Check sheet for the modelled part. Datum: model origin and axes. Units: mm. A direction names the side the tool comes from. Coordinates: 2 decimals unless noted, no trailing zeros. Write each loop counter-clockwise with the first axis right and the second up, starting at its lowest first coordinate (ties: lowest second). Pieces come first, ordered by that corner, then holes. Notation, with made-up numbers: (-1.5, 63.5) - (10.5, 63.5) arc R36 cw to (10.5, 101.5) - close; hole circle Ø11 at (73, 88.25). An arc over 180 degrees is marked (long way). Answer as CSV lines item,"result". Start each with the question number.
Autodesk Inventor part; units mm, degrees
ref_plane "YZ Plane" through (0, 0, 0) normal (1, 0, 0) x (0, 1, 0)
ref_plane "XZ Plane" through (0, 0, 0) normal (0, 1, 0) x (-1, 0, 0)
ref_plane "XY Plane" through (0, 0, 0) normal (0, 0, 1) x (1, 0, 0)
sketch "スケッチ1" plane through (0, 0, 0) normal (0, 0, 1) x (1, 0, 0)
  line L0 (-28, 65) -> (28, 65)
  line L1 (28, 65) -> (28, 47.1)
  line L2 (-28, -65) -> (-28, -47.1)
  line L3 (-28, 65) -> (28, -65) construction
  line L4 (28, 65) -> (-28, -65) construction
  line L5 (-28, 45) -> (-33, 45)
  line L6 (-33, 15) -> (-28, 15)
  line L7 (-33, 15) -> (-33, 45)
  line L8 (-28, -15) -> (-33, -15)
  line L9 (-33, -15) -> (-33, -45)
  line L10 (-33, -45) -> (-28, -45)
  arc A0 (-28, 45) -> (-28, 47.1) centre (-28, 46.05) ccw
  arc A1 (-28, 12.9) -> (-28, 15) centre (-28, 13.95) ccw
  arc A2 (-28, -15) -> (-28, -12.9) centre (-28, -13.95) ccw
  arc A3 (-28, -47.1) -> (-28, -45) centre (-28, -46.05) ccw
  line L11 (-28, 47.1) -> (-28, 65)
  line L12 (-28, 12.9) -> (-28, 15) construction
  line L13 (-28, -12.9) -> (-28, 12.9)
  line L14 (-28, -47.1) -> (-28, -45) construction
  line L15 (0, 65) -> (0, -65) construction
  arc A4 (28, -45) -> (28, -47.1) centre (28, -46.05) ccw
  line L16 (33, -45) -> (28, -45)
  line L17 (33, -15) -> (33, -45)
  line L18 (28, -15) -> (33, -15)
  arc A5 (28, -12.9) -> (28, -15) centre (28, -13.95) ccw
  arc A6 (28, 15) -> (28, 12.9) centre (28, 13.95) ccw
  line L19 (33, 15) -> (33, 45)
  line L20 (33, 15) -> (28, 15)
  line L21 (28, 45) -> (33, 45)
  arc A7 (28, 47.1) -> (28, 45) centre (28, 46.05) ccw
  line L22 (28, 47.1) -> (28, 45) construction
  line L23 (28, 12.9) -> (28, -12.9)
  line L24 (28, -47.1) -> (28, -65)
  line L25 (28, -12.9) -> (28, -15) construction
  line L26 (-28, -15) -> (-28, -12.9) construction
  line L27 (-28, -45) -> (-28, -15)
  line L28 (28, -15) -> (28, -45)
  line L29 (28, -45) -> (28, -47.1) construction
  line L30 (-20, -25) -> (-15, -25) construction
  line L31 (-15, -25) -> (-15, -45) construction
  line L32 (-15, -45) -> (-20, -45) construction
  line L33 (-20, -45) -> (-20, -25) construction
  line L34 (-20, -25) -> (-15, -45) construction
  line L35 (-15, -25) -> (-20, -45) construction
  line L36 (-20, 2.5) -> (-15, 2.5) construction
  line L37 (-15, 2.5) -> (-15, -72.5) construction
  line L38 (-15, -72.5) -> (-20, -72.5) construction
  line L39 (-20, -72.5) -> (-20, 2.5) construction
  line L40 (-20, 2.5) -> (-15, -72.5) construction
  line L41 (-15, 2.5) -> (-20, -72.5) construction
  circle A8 centre (-17.5, -55) radius 1.55
  line L42 (-20, -35) -> (-15, -35) construction
  line L43 (-17.5, 2.5) -> (-17.5, -72.5) construction
  circle A9 centre (-17.5, -15) radius 1.55
  circle A10 centre (17.5, -55) radius 1.55
  circle A11 centre (17.5, -15) radius 1.55
  line L44 (28, -65) -> (12.5, -65) construction
  line L45 (-12.5, -62.5) -> (-12.5, -45)
  line L46 (-12.5, -45) -> (0, -45)
  line L47 (12.5, -62.5) -> (12.5, -45)
  line L48 (12.5, -45) -> (0, -45)
  line L49 (-12.5, -65) -> (-28, -65) construction
  line L50 (12.5, -65) -> (-12.5, -65) construction
  line L51 (-28, 45) -> (-28, 47.1) construction
  line L52 (-28, 15) -> (-28, 45)
  line L53 (28, 15) -> (28, 12.9) construction
  line L54 (28, 45) -> (28, 15)
  circle A12 centre (-24.5, 43.5) radius 1.25
  line L55 (-28, 0) -> (28, 0) construction
  line L56 (-28, 46.5) -> (28, 46.5) construction
  circle A13 centre (-24.5, -61.5) radius 1.25
  circle A14 centre (24.5, 43.5) radius 1.25
  circle A15 centre (24.5, -61.5) radius 1.25
  circle A16 centre (-17.5, -55) radius 3 construction
  line L57 (-12.5, -62.5) -> (12.5, -62.5)
  line L58 (-20, 41.5) -> (20, 41.5)
  line L59 (20, 2.5) -> (-20, 2.5)
  line L60 (-20, 2.5) -> (-20, 41.5)
  line L61 (20, 2.5) -> (20, 41.5)
  line L62 (-20.05, -43.5651) -> (-18.5651, -45.05) construction
  line L63 (-19.3075, -44.3075) -> (-20.05, -45.05) construction
  arc A17 (-20.05, -43.5651) -> (-18.5651, -45.05) centre (-19.3075, -44.3075) ccw
  line L64 (-20.05, -24.95) -> (-18.5651, -24.95) construction
  line L65 (-14.95, -24.95) -> (-14.95, -26.4349) construction
  line L66 (-14.95, -45.05) -> (-16.4349, -45.05) construction
  line L67 (-20.05, -45.05) -> (-20.05, -43.5651) construction
  line L68 (-20.05, -24.95) -> (-14.95, -45.05) construction
  line L69 (-14.95, -24.95) -> (-20.05, -45.05) construction
  arc A18 (-16.4349, -45.05) -> (-14.95, -43.5651) centre (-15.6925, -44.3075) ccw
  arc A19 (-18.5651, -24.95) -> (-20.05, -26.4349) centre (-19.3075, -25.6925) ccw
  arc A20 (-14.95, -26.4349) -> (-16.4349, -24.95) centre (-15.6925, -25.6925) ccw
  line L70 (-20.05, -43.5651) -> (-20.05, -26.4349)
  line L71 (-18.5651, -45.05) -> (-20.05, -45.05) construction
  line L72 (-16.4349, -45.05) -> (-18.5651, -45.05)
  line L73 (-14.95, -43.5651) -> (-14.95, -45.05) construction
  line L74 (-20.05, -26.4349) -> (-20.05, -24.95) construction
  line L75 (-18.5651, -24.95) -> (-16.4349, -24.95)
  line L76 (-16.4349, -24.95) -> (-14.95, -24.95) construction
  line L77 (-14.95, -26.4349) -> (-14.95, -43.5651)
  arc A21 (18.5651, -45.05) -> (20.05, -43.5651) centre (19.3075, -44.3075) ccw
  arc A22 (14.95, -43.5651) -> (16.4349, -45.05) centre (15.6925, -44.3075) ccw
  arc A23 (16.4349, -24.95) -> (14.95, -26.4349) centre (15.6925, -25.6925) ccw
  arc A24 (20.05, -26.4349) -> (18.5651, -24.95) centre (19.3075, -25.6925) ccw
  line L78 (20.05, -43.5651) -> (20.05, -26.4349)
  line L79 (16.4349, -45.05) -> (18.5651, -45.05)
  line L80 (18.5651, -24.95) -> (16.4349, -24.95)
  line L81 (14.95, -26.4349) -> (14.95, -43.5651)
  line L82 (-28, -65) -> (-28, -70)
  line L83 (-28, -70) -> (28, -70)
  line L84 (28, -70) -> (28, -65)
  point P0 (0, 0)
  point P1 (0, 0)
  point P2 (0, 0)
  point P3 (28, 45)
  point P4 (-17.5, -35)
  point P5 (28, 45)
  dimension "d0" = 56
  dimension "d1" = 130
  dimension "d2" = 20
  dimension "d3" = 30
  dimension "d4" = 30
  dimension "d5" = 30
  dimension "d6" = 1.05
  dimension "d7" = 1.05
  dimension "d8" = 1.05
  dimension "d9" = 1.05
  dimension "d10" = 5
  dimension "d23" = 15
  dimension "d24" = 5
  dimension "d25" = 20
  dimension "d28" = 3.1
  dimension "d72" = 75
  dimension "d94" = 20
  dimension "d103" = 8
  dimension "d109" = 80
  dimension "d111" = 20
  dimension "d113" = 3.5
  dimension "d114" = 2.5
  dimension "d115" = 18.5
  dimension "d116" = 3
  dimension "d117" = 2.5
  dimension "d118" = 3.5
  dimension "d119" = 3.5
  dimension "d120" = 25
  dimension "d121" = 6
  dimension "d124" = 2.5
  dimension "d125" = 7.5
  dimension "d126" = 8
  dimension "d128" = 5
  dimension "d130" = 1.05
  dimension "d131" = 0.05
  dimension "d132" = 0.05
  dimension "d133" = 5
extrude "押し出し1" add sketch "スケッチ1" along normal blind 2.5
extrude "押し出し2" add sketch "スケッチ1" along normal blind 5 contours L0 L1 A7 L54 A6 L23 A5 L28 A4 L24 L84 L83 L82 L2 A3 L27 A2 L13 A1 L52 A0 L11
fillet "フィレット1" radius 1 7 edges at (-12.5, -45, 2.5) (-12.5, -62.5, 2.5) (12.5, -62.5, 2.5) (-20, 41.5, 2.5) (20, 41.5, 2.5) (20, 2.5, 2.5) (-20, 2.5, 2.5)
sketch "スケッチ7" plane through (28, -70, 0) normal (1, 0, 0) x (0, 0, -1)
  line L0 (0, 55) -> (-2.5, 55)
  line L1 (0, 57.1) -> (0, 82.9)
  line L2 (0, 0) -> (0, 22.9)
  point P0 (0, 70)
  point P1 (-2.5, 15)
  point P2 (-2.5, 65)
  point P3 (0, 25)
  dimension "d136" = 10
  dimension "d137" = 10
  dimension "d138" = 2.5
  dimension "d139" = 2.5
hole "穴6" at (28, -55, 2.5) at (28, -5, 2.5) direction (-1, 0, 0) diameter 2.459 depth 4
sketch "スケッチ8" plane through (-28, -70, 0) normal (-1, 0, 0) x (0, 0, 1)
  circle A0 centre (2.5, 15) radius 1.2295
  circle A1 centre (2.5, 65) radius 1.2295
  point P0 (0, 70)
hole "穴7" at (-28, -5, 2.5) at (-28, -55, 2.5) direction (1, 0, 0) diameter 2.459 depth 4
equation "\"d2\" = -0.5 * d4 + 0.5 * d1 - d3"
equation "\"d5\" = d3"
equation "\"d7\" = d6"
equation "\"d8\" = d7"
equation "\"d9\" = d8"
properties part number "Cockpit_horizontal_frame_02" material "アセタール樹脂、黒"
(1) Cross-section at B-B on y = -55. Record the boundary of the cut face in (x, z), plus the area to 3 significant figures.
(2) Tool access check on faces 4 (the face through (-31, 15, 1)), 5 (the face through (30, -15, 1)), 6 (the face through (-24, -55, 2)), 7 (the face through (30, 30, 2.5)). Record the directions out of +Z, -Z, +X, -X, +Y, -Y that give a thin tool (end or side, any length) a straight path to the whole face; none if there is none.
(3) Cross-section at A-A on y = 37. Record the boundary of the cut face in (x, z).
(4) Go/stop test with flat-tipped pins: P1, Ø2, axis at x = -24.5, y = -61.5, coming from the +Z side; P2, Ø1.2, axis at x = 30, z = 1, coming from the -Y side; P3, Ø1, axis at y = 40.5, z = 3.5, coming from the +X side; P4, Ø1.5, axis at y = -5, z = 2.5, coming from the -X side. Record where each tip stops, or that it passes through.
(5) Material ranges on probe 1 along Y at (x, z) = (17.5, 1.7); probe 2 along Y at (x, z) = (-8.5, 2.75); probe 3 along Y at (x, z) = (29, 1.4), recorded low to high. Write a range as from..to.
(6) Release check for a two-part mould opening along X. For faces 1 (the face through (12.5, -53, 2)), 2 (the face through (25.97, -3.91, 1.93)), 3 (the face through (33, 30, 1)) record: pulls with the +X half, pulls with the -X half, needs draft (parallel to the pull), parting line crosses it, or undercut.
(7) Cross-section at C-C on x = -1. Record the boundary of the cut face in (y, z).
Checked values:
1,outline,"(-28, 0) - (-19.05, 0) - (-19.05, 5) - (-28, 5) - (-28, 3.73) - (-24, 3.73) - (-24, 1.27) - (-28, 1.27) - close; (-15.95, 0) - (-12.5, 0) - (-12.5, 5) - (-15.95, 5) - close; (12.5, 0) - (15.95, 0) - (15.95, 5) - (12.5, 5) - close; (19.05, 0) - (28, 0) - (28, 1.27) - (24, 1.27) - (24, 3.73) - (28, 3.73) - (28, 5) - (19.05, 5) - close"
1,area,"104 mm^2"
2,face 4,"+Z, -Z, -X"
2,face 5,"+Z, -Z, +X"
2,face 6,"-X"
2,face 7,"+Z, +X, +Y, -Y"
3,outline,"(-33, 0) - (-20, 0) - (-20, 5) - (-28, 5) - (-28, 2.5) - (-33, 2.5) - close; (20, 0) - (33, 0) - (33, 2.5) - (28, 2.5) - (28, 5) - (20, 5) - close"
4,P1,"through"
4,P2,"y = -45"
4,P3,"x = 28"
4,P4,"x = -24"
5,probe 1,"-70..-56.55, -53.45..-45.05, -24.95..-16.55, -13.45..2.5, 41.5..65"
5,probe 2,"-70..-62.5, -45..2.5, 41.5..65"
5,probe 3,"-45..-15, 15..45"
6,face 1,"undercut"
6,face 2,"needs draft"
6,face 3,"pulls with the +X half"
7,outline,"(-70, 0) - (-62.5, 0) - (-62.5, 5) - (-70, 5) - close; (-45, 0) - (2.5, 0) - (2.5, 5) - (-45, 5) - close; (41.5, 0) - (65, 0) - (65, 5) - (41.5, 5) - close"
